```python
from build123d import *


with BuildPart() as part:
    # Sketch1 → Revolve1 (revolve)
    with BuildSketch(Plane.XZ.offset(-22), mode=Mode.PRIVATE) as revolve1_sk:
        with BuildLine():
            Line((5, 2.5), (5, -2.5))
            ThreePointArc((5, -2.5), (5.146446609, -2.853553391), (5.5, -3))
            Line((5.5, -3), (10.5, -3))
            ThreePointArc((10.5, -3), (10.853553391, -2.853553391), (11, -2.5))
            Line((11, -2.5), (11, 2.5))
            ThreePointArc((11, 2.5), (10.853553391, 2.853553391), (10.5, 3))
            Line((10.5, 3), (8.75, 3))
            Line((8.75, 3), (8.75, -1.5))
            Line((8.75, -1.5), (7.25, -1.5))
            Line((7.25, -1.5), (7.25, 3))
            Line((7.25, 3), (5.5, 3))
            ThreePointArc((5.5, 3), (5.146446609, 2.853553391), (5, 2.5))
        make_face()
    revolve(revolve1_sk.sketch.rotate(Axis((0, 22, 3), (0, 0, -1)), 180), axis=Axis((0, 22, 3), (0, 0, -1)))


solid = part.part
```
Work out the finished part from the listing and answer in its coordinate system (mm). A direction names the side the tool comes from. Round coordinates to 2 decimals unless told otherwise and drop trailing zeros. Order: outer loops, then holes, each group sorted by start corner. A loop starts at its lowest first (then second) coordinate and runs counter-clockwise, first axis right, second up.
Q1. A cutting plane is placed at A-A, the plane y = 22. Determine the outline of the cut face in (x, z).
Solution:
outline: (-11, -2.5) arc R0.5 ccw to (-10.5, -3) - (-5.5, -3) arc R0.5 ccw to (-5, -2.5) - (-5, 2.5) arc R0.5 ccw to (-5.5, 3) - (-7.25, 3) - (-7.25, -1.5) - (-8.75, -1.5) - (-8.75, 3) - (-10.5, 3) arc R0.5 ccw to (-11, 2.5) - close; (5, -2.5) arc R0.5 ccw to (5.5, -3) - (10.5, -3) arc R0.5 ccw to (11, -2.5) - (11, 2.5) arc R0.5 ccw to (10.5, 3) - (8.75, 3) - (8.75, -1.5) - (7.25, -1.5) - (7.25, 3) - (5.5, 3) arc R0.5 ccw to (5, 2.5) - close
Q2. The mould has two halves that part along Y. Classify faces 1 (the flat face through (3, 29, -1.5)), 2 (the cylindrical face through (2.38, 11.26, 0.04)), 3 (the cylindrical face through (1.08, 17.12, -0.04)), 4 (the flat face through (-3, 27, 3)): pulls with the +Y half, pulls with the -Y half, needs draft (parallel to the pull), parting line crosses it, or undercut.
Solution:
face 1: undercut
face 2: parting line crosses it
face 3: undercut
face 4: needs draft
Q3. A tool of negligible diameter and unlimited length cuts with its end or side. For faces 5 (the cylindrical face through (6.45, 27.91, 0.72)), 6 (the flat face through (5, 17, -3)), from which of +Z, -Z, +X, -X, +Y, -Y can it reach the whole face along a straight path? Write none if from no direction.
Solution:
face 5: +Z
face 6: -Z, +X, -X, +Y, -Y
Q4. Given pin 1 Ø1 at (x, z) = (-1.5, -1.5) entering from +Y, flat-ended and moving along its own axis, determine where the tip first touches the part or whether it passes through.
Solution:
pin 1: stops at y = 32.95
Q5. A cutting plane is placed at C-C, the plane z = -0.25. Determine the outline of the cut face in (x, y), then the cut area to 3 significant figures.
Solution:
outline: circle Ø22 at (0, 22); circle Ø14.5 at (0, 22); hole circle Ø17.5 at (0, 22); hole circle Ø10 at (0, 22)
area: 226 mm2
Q6. A cutting plane is placed at B-B, the plane x = 0. Determine the outline of the cut face in (y, z).
Solution:
outline: (11, -2.5) arc R0.5 ccw to (11.5, -3) - (16.5, -3) arc R0.5 ccw to (17, -2.5) - (17, 2.5) arc R0.5 ccw to (16.5, 3) - (14.75, 3) - (14.75, -1.5) - (13.25, -1.5) - (13.25, 3) - (11.5, 3) arc R0.5 ccw to (11, 2.5) - close; (27, -2.5) arc R0.5 ccw to (27.5, -3) - (32.5, -3) arc R0.5 ccw to (33, -2.5) - (33, 2.5) arc R0.5 ccw to (32.5, 3) - (30.75, 3) - (30.75, -1.5) - (29.25, -1.5) - (29.25, 3) - (27.5, 3) arc R0.5 ccw to (27, 2.5) - close
Q7. Find the intervals of material crossed by line 1 along Y through (x, z) = (0.25, -1.25); line 2 along X through (y, z) = (21.75, 1.75); line 3 along Y through (x, z) = (-2.75, 2.5), in increasing order.
Solution:
line 1: y = 11 to 13.25, 14.75 to 17.01, 26.99 to 29.25, 30.75 to 33
line 2: x = -11 to -8.75, -7.25 to -4.99, 4.99 to 7.25, 8.75 to 11
line 3: y = 11.35 to 13.69, 15.29 to 17.82, 26.18 to 28.71, 30.31 to 32.65
